from build123d import *

# Parameters (mm, degrees)
SKETCH018_W     = 151.632408
SKETCH018_H     = 21.2714
PAD011_DEPTH    = 40
SKETCH019_W     = 121.632408
SKETCH019_H     = 24
POCKET007_DEPTH = 21.2724
FILLET010_R     = 15
FILLET011_R     = 5


with BuildPart() as part:
    # Sketch018 (on Face1 of CopyPocket006) → Pad011 (new body)
    with BuildSketch(Plane.XZ.offset(825)):
        with Locations((-597.5, -869.507206)):
            Rectangle(SKETCH018_W, SKETCH018_H)
    extrude(amount=PAD011_DEPTH)

    # Sketch019 (on Face4 of Pad011) → Pocket007 (cut, through all)
    with BuildSketch(Plane(origin=(0, 0, -858.871506), x_dir=(-1, 0, 0), z_dir=(0, 0, 1))):
        with Locations((597.5, 838)):
            Rectangle(SKETCH019_W, SKETCH019_H)
    extrude(amount=-POCKET007_DEPTH, mode=Mode.SUBTRACT)

    # Fillet010
    fillet010_edges = [part.edges().sort_by_distance(p)[0] for p in [
        (-673.316204, -865, -869.507206),
        (-521.683796, -865, -869.507206),
        (-658.316204, -850, -869.507206),
        (-536.683796, -850, -869.507206),
    ]]
    fillet(fillet010_edges, radius=FILLET010_R)

    # Fillet011
    fillet011_edges = [part.edges().sort_by_distance(p)[0] for p in [
        (-597.5, -850, -858.871506),
        (-597.5, -850, -880.142906),
        (-597.5, -865, -858.871506),
        (-597.5, -865, -880.142906),
    ]]
    fillet(fillet011_edges, radius=FILLET011_R)


solid = part.part
Work out the finished part from the listing and answer in its coordinate system (mm). A direction names the side the tool comes from. Give positions to 0.01 mm unless a question says otherwise; leave off trailing zeros. Order: outer loops, then holes, each group sorted by start corner. A loop starts at its lowest first (then second) coordinate and runs counter-clockwise, first axis right, second up. Notation, with made-up numbers: (49.5, 85) -> (103.5, 85) arc R8 ccw to (103.5, 93) -> close; hole circle Ø1 at (53, 6). An arc over 180 degrees is marked (long way). One line per item, written item: value.
Item 1: Find section B-B, the plane x = -605. Give the vertices of the cut face in (y, z).
Answer sheet:
outline: (-865, -875.14) arc R5 ccw to (-860, -880.14) -> (-855, -880.14) arc R5 ccw to (-850, -875.14) -> (-850, -863.87) arc R5 ccw to (-855, -858.87) -> (-860, -858.87) arc R5 ccw to (-865, -863.87) -> close; (-826, -880.14) -> (-825, -880.14) -> (-825, -858.87) -> (-826, -858.87) -> close
Item 2: Find section C-C, the plane y = -829.5. Give the vertices of the cut face in (x, z).
Answer sheet:
outline: (-673.32, -875.14) arc R5 ccw to (-668.32, -880.14) -> (-663.32, -880.14) arc R5 ccw to (-658.32, -875.14) -> (-658.32, -863.87) arc R5 ccw to (-663.32, -858.87) -> (-668.32, -858.87) arc R5 ccw to (-673.32, -863.87) -> close; (-536.68, -875.14) arc R5 ccw to (-531.68, -880.14) -> (-526.68, -880.14) arc R5 ccw to (-521.68, -875.14) -> (-521.68, -863.87) arc R5 ccw to (-526.68, -858.87) -> (-531.68, -858.87) arc R5 ccw to (-536.68, -863.87) -> close
Item 3: Straight lines are drawn through the part: probe 1 along Y at (x, z) = (-613, -869); probe 2 along X at (y, z) = (-845, -874); probe 3 along Y at (x, z) = (-582.5, -860.75). For each, find the intervals that lie inside material, in ascending order.
Answer sheet:
probe 1: -865 to -850, -826 to -825
probe 2: -673.32 to -654.5, -540.5 to -521.68
probe 3: -863.91 to -851.09, -826 to -825
Item 4: Find section A-A, the plane z = -866.25. Give the vertices of the cut face in (x, y).
Answer sheet:
outline: (-673.32, -850) arc R15 ccw to (-658.32, -865) -> (-536.68, -865) arc R15 ccw to (-521.68, -850) -> (-521.68, -825) -> (-673.32, -825) -> close; hole (-658.32, -835) arc R15 ccw to (-643.32, -850) -> (-551.68, -850) arc R15 ccw to (-536.68, -835) -> (-536.68, -826) -> (-658.32, -826) -> close
Item 5: A tool of negligible diameter and unlimited length cuts with its end or side. For faces 1 (the flat face through (-597.8, -855.4, -880.143)), 2 (the cylindrical face through (-654.04, -845.49, -869.59)), 3 (the cylindrical face through (-598.1, -851.5, -860.3)), 4 (the cylindrical face through (-596.649, -863.496, -878.717)), 5 (the cylindrical face through (-535.2, -830.6, -878.7)), from which of +Z, -Z, +X, -X, +Y, -Y can it reach the whole face along a straight path? Write none if from no direction.
Answer sheet:
face 1: -Z, +X, -X, +Y, -Y
face 2: +Z, -Z
face 3: +Z
face 4: -Z, +X, -X, -Y
face 5: -Z
Item 6: Flat-ended cylindrical pins translate along their axes: P1, Ø2, axis at y = -861, z = -866, coming from the -X side; P2, Ø6, axis at y = -855.5, z = -863.5, coming from the +X side. Find the tip coordinate at first contact, or state that the pin passes through.
Answer sheet:
P1: x = -669.5
P2: x = -521.9
Item 7: Determine the mould class of faces 6 (the flat face through (-673.316, -837, -870)), 7 (the cylindrical face through (-535.18, -830.563, -860.297)), 8 (the cylindrical face through (-526.19, -860.72, -869.43)), 9 (the cylindrical face through (-541.19, -845.72, -869.59)) for opening direction Y: released by +Y, released by -Y, zero draft, split by the parting line, or undercut.
Answer sheet:
face 6: zero draft
face 7: undercut
face 8: released by -Y
face 9: undercut
